Source: CAD feature listing. Evaluate the final solid. Frame: model axes, mm. A direction names the side the tool comes from. Round coordinates to 2 decimals unless told otherwise and drop trailing zeros. Order: outer loops, then holes, each group sorted by start corner. A loop starts at its lowest first (then second) coordinate and runs counter-clockwise, first axis right, second up. Notation, with made-up numbers: (83.5, 5.5) -> (107.5, 5.5) arc R15 cw to (107.5, 26.5) -> close; hole circle Ø4 at (89.25, 75). An arc over 180 degrees is marked (long way). Answer as CSV lines item,"result".
from build123d import *

# Parameters (mm, degrees)
F0_W     = 1745.899328
F0_H     = 1752.6
F1_DEPTH = 728.98
F2_R     = 266.7
F3_DEPTH = 949.96
F4_W     = 1473.042846
F4_H     = 545.412392
F4_R     = 331.059319
F5_DEPTH = 1889.76


with BuildPart() as f1:
    # F0 (on Right) → F1 (new body)
    with BuildSketch(Plane.YZ):
        Rectangle(F0_W, F0_H)
    extrude(amount=F1_DEPTH)

    # F2 (on face) → F3 (cut)
    with BuildSketch(Plane.YZ.offset(728.98)):
        with Locations((-427.558064, 463.162661)):
            Circle(F2_R)
    extrude(amount=-F3_DEPTH, mode=Mode.SUBTRACT)

    # F4 (on face) → F5 (cut)
    with BuildSketch(Plane.YZ.offset(728.98)):
        with Locations((0, -432.679504)):
            Rectangle(F4_W, F4_H)
        with Locations((485.288173, 447.710544)):
            Circle(F4_R)
    extrude(amount=-F5_DEPTH, mode=Mode.SUBTRACT)


solid = f1.part
1. Mould query, pull axis Y, two halves, no side actions, for faces 3 (the flat face through (370, -10, -705.386)), 4 (the flat face through (728.98, -12, 12)), 5 (the flat face through (370, -736.521, -436)), 6 (the flat face through (359, 872.95, -12)). Classes: released by +Y, released by -Y, zero draft, split by the parting line, or undercut.
Results below:
face 3,"undercut"
face 4,"zero draft"
face 5,"undercut"
face 6,"released by +Y"
2. Line query: L1, parallel to Z at x = 440.5, y = 493; L2, parallel to Z at x = 570.5, y = 624; L3, parallel to Y at x = 528, z = -441.5. Output: solid intervals per line, ascending. Write a range as [from, to].
Results below:
L1,"[-876.3, -705.39], [-159.97, 116.74], [778.68, 876.3]"
L2,"[-876.3, -705.39], [-159.97, 147.11], [748.31, 876.3]"
L3,"[-872.95, -736.52], [736.52, 872.95]"
3. Section query D-D on x = 528. Return loops of the section in (y, z), and give its area (3 significant figures).
Results below:
outline,"(-872.95, -876.3) -> (872.95, -876.3) -> (872.95, 876.3) -> (-872.95, 876.3) -> close; hole (-736.52, -705.39) -> (736.52, -705.39) -> (736.52, -159.97) -> (-736.52, -159.97) -> close; hole circle Ø533.4 at (-427.56, 463.16); hole circle Ø662.12 at (485.29, 447.71)"
area,"1,690,000 mm2"
4. Section query A-A on z = -494. Return loops of the section in (x, y), and give its area (3 significant figures).
Results below:
outline,"(0, -872.95) -> (728.98, -872.95) -> (728.98, -736.52) -> (0, -736.52) -> close; (0, 736.52) -> (728.98, 736.52) -> (728.98, 872.95) -> (0, 872.95) -> close"
area,"199,000 mm2"
5. Section query B-B on y = -131.5. Return loops of the section in (x, z), and give its area (3 significant figures).
Results below:
outline,"(0, -876.3) -> (728.98, -876.3) -> (728.98, -705.39) -> (0, -705.39) -> close; (0, -159.97) -> (728.98, -159.97) -> (728.98, 876.3) -> (0, 876.3) -> close"
area,"880,000 mm2"
6. Section query C-C on z = 421.5. Return loops of the section in (x, y), and give its area (3 significant figures).
Results below:
outline,"(0, -872.95) -> (728.98, -872.95) -> (728.98, -690.98) -> (0, -690.98) -> close; (0, -164.13) -> (728.98, -164.13) -> (728.98, 155.27) -> (0, 155.27) -> close; (0, 815.31) -> (728.98, 815.31) -> (728.98, 872.95) -> (0, 872.95) -> close"
area,"408,000 mm2"
7. Reachability of faces 1 (the flat face through (359, -872.95, -12)), 2 (the flat face through (370, -10, -159.973)) from +Z, -Z, +X, -X, +Y, -Y: full face, straight path, thin tool, end or side. Return the list, or none.
Results below:
face 1,"+Z, -Z, +X, -X, -Y"
face 2,"+X, -X"
